Could you check a few things on this model? Use its own coordinates, in mm. Coordinates: 2 decimals unless noted, no trailing zeros. Write each loop counter-clockwise with the first axis right and the second up, starting at its lowest first coordinate (ties: lowest second). Pieces come first, ordered by that corner, then holes. Notation, with made-up numbers: (68.25, 56) - (99.25, 56) arc R13 ccw to (99.25, 72) - close; hole circle Ø3 at (-16.75, 78.5). An arc over 180 degrees is marked (long way). Write item = value, one per line. Start each with the question number.
```python
from build123d import *

# Parameters (mm, degrees)
SKETCH_1_W          = 5
SKETCH_1_H          = 60
SKETCH_1_W_2        = 30
SKETCH_1_H_2        = 5
SKETCH_1_W_3        = 15
EXTRUDE_1_DEPTH     = 5
FILLET_1_R          = 5
SKETCH_2_W          = 245
SKETCH_2_H          = 125
CUT_EXTRUDE_1_DEPTH = 5
SKETCH_3_W          = 110
SKETCH_3_H          = 2.5
SKETCH_3_W_2        = 115
CUT_EXTRUDE_2_DEPTH = 10
SKETCH_4_W          = 5
SKETCH_4_H          = 5
CUT_EXTRUDE_3_DEPTH = 5


with BuildPart() as part:
    # 草圖1 → 填料-伸長1 (new body)
    with BuildSketch(Plane(origin=(0, 0, 0), x_dir=(1, 0, 0), z_dir=(0, 1, 0))):
        Polygon((198.746286718, -286.464902661), (198.746286718, -256.464902661), (183.246286718, -256.464902661), (183.246286718, -266.464902661), (124.746286718, -266.464902661), (124.746286718, -262.464902661), (109.246286718, -262.464902661), (109.246286718, -266.464902661), (-21.253713282, -266.464902661), (-21.253713282, 38.535097339), (-36.253713282, 38.535097339), (-36.253713282, 43.535097339), (203.746286718, 43.535097339), (203.746286718, -286.464902661), align=None)
        with Locations((206.246286718, -256.464902661)):
            Rectangle(SKETCH_1_W, SKETCH_1_H)
        with Locations((206.246286718, 13.535097339)):
            Rectangle(SKETCH_1_W, SKETCH_1_H)
        with Locations((188.746286718, 46.035097339)):
            Rectangle(SKETCH_1_W_2, SKETCH_1_H_2)
        with Locations((-21.253713282, 46.035097339)):
            Rectangle(SKETCH_1_W_2, SKETCH_1_H_2)
        with Locations((91.246286718, 46.035097339)):
            Rectangle(SKETCH_1_W_3, SKETCH_1_H_2)
        with Locations((76.246286718, 46.035097339)):
            Rectangle(SKETCH_1_W_3, SKETCH_1_H_2)
        with Locations((206.246286718, -166.464902661)):
            Rectangle(SKETCH_1_W, SKETCH_1_H)
        with Locations((206.246286718, -76.464902661)):
            Rectangle(SKETCH_1_W, SKETCH_1_H)
    extrude(amount=EXTRUDE_1_DEPTH)

    # 圓角1
    fillet_1_edges = [part.edges().sort_by_distance(p)[0] for p in [
        (208.746286718, 5, -13.535097339),
        (208.746286718, 5, 76.464902661),
        (208.746286718, 5, 166.464902661),
        (208.746286718, 5, 256.464902661),
    ]]
    fillet(fillet_1_edges, radius=FILLET_1_R - 0.0001)  # a hair under: the kernel refuses the full size

    # 草圖2 → 除料-伸長1 (cut)
    with BuildSketch(Plane(origin=(0, 5, 0), x_dir=(1, 0, 0), z_dir=(0, 1, 0))):
        with Locations((86.246286718, -13.964902661)):
            Rectangle(SKETCH_2_W, SKETCH_2_H)
    extrude(amount=-CUT_EXTRUDE_1_DEPTH, mode=Mode.SUBTRACT)

    # 草圖3 → 除料-伸長2 (cut)
    with BuildSketch(Plane(origin=(0, 0, 76.464902661), x_dir=(-1, 0, 0), z_dir=(0, 0, -1))):
        with Locations((-33.746286718, 1.25)):
            Rectangle(SKETCH_3_W, SKETCH_3_H)
        with Locations((-151.246286718, 3.75)):
            Rectangle(SKETCH_3_W_2, SKETCH_3_H)
    extrude(amount=-CUT_EXTRUDE_2_DEPTH, mode=Mode.SUBTRACT)

    # 草圖4 → 除料-伸長3 (cut)
    with BuildSketch(Plane(origin=(0, 0, 76.464902661), x_dir=(-1, 0, 0), z_dir=(0, 0, -1))):
        with Locations((-91.246286718, 2.5)):
            Rectangle(SKETCH_4_W, SKETCH_4_H)
    extrude(amount=-CUT_EXTRUDE_3_DEPTH, mode=Mode.SUBTRACT)


solid = part.part
```
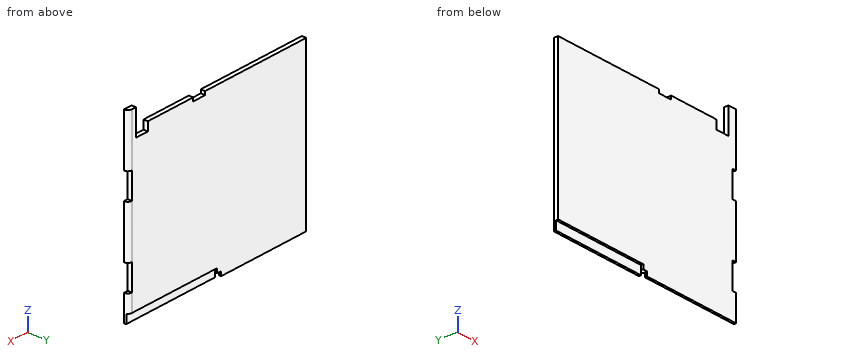
1) For P1, Ø3, axis at y = 0.5, z = 215.5, coming from the +X side; P2, Ø2.5, axis at y = 3.5, z = 263.5, coming from the +X side; P3, Ø0.8, axis at y = 1.5, z = 84, coming from the -X side; P4, Ø5, axis at x = 32.5, z = 237.5, coming from the -Y side, each with a flat end and sliding along its axis, tell me the tip position at first contact or that it passes through.
2) Suppose I cut it at A-A on y = 1.55. Please give me the cut outline in (x, z), plus the area to 3 significant figures.
3) Suppose I cut it at B-B on x = 27. Please give me the cut outline in (y, z), plus the area to 3 significant figures.
4) If I drill on probe 1 along Z at (x, y) = (151.5, 0.8); probe 2 along X at (y, z) = (0.5, 246); probe 3 along X at (y, z) = (0.9, 119), over which ranges is the centre line in solid material (lowest first)? Write a range as [from, to].
5) Suppose I cut it at C-C on z = 129.5. Please give me the cut outline in (x, y), plus the area to 4 significant figures.
6) Suppose I cut it at D-D on x = 192. Please give me the cut outline in (y, z), plus the area to 3 significant figures.
Reply:
q1.P1 = 203.75
q1.P2 = 208.21
q1.P3 = 88.75
q1.P4 = 0
q2.outline = (-21.25, 86.46) - (88.75, 86.46) - (88.75, 81.46) - (93.75, 81.46) - (93.75, 76.46) - (208.5, 76.46) - (208.5, 106.46) - (203.75, 106.46) - (203.75, 136.46) - (208.5, 136.46) - (208.5, 196.46) - (203.75, 196.46) - (203.75, 226.46) - (208.5, 226.46) - (208.5, 286.46) - (198.75, 286.46) - (198.75, 256.46) - (183.25, 256.46) - (183.25, 266.46) - (124.75, 266.46) - (124.75, 262.46) - (109.25, 262.46) - (109.25, 266.46) - (-21.25, 266.46) - close
q2.area = 42,200 mm^2
q3.outline = (0, 86.46) - (2.5, 86.46) - (2.5, 76.46) - (5, 76.46) - (5, 266.46) - (0, 266.46) - close
q3.area = 925 mm^2
q4.probe_1 = [76.46, 266.46]
q4.probe_2 = [-21.25, 208.72]
q4.probe_3 = [-21.25, 203.75]
q5.outline = (-21.25, 0) - (203.75, 0) - (203.75, 5) - (-21.25, 5) - close
q5.area = 1,125 mm^2
q6.outline = (0, 76.46) - (2.5, 76.46) - (2.5, 86.46) - (5, 86.46) - (5, 256.46) - (0, 256.46) - close
q6.area = 875 mm^2
